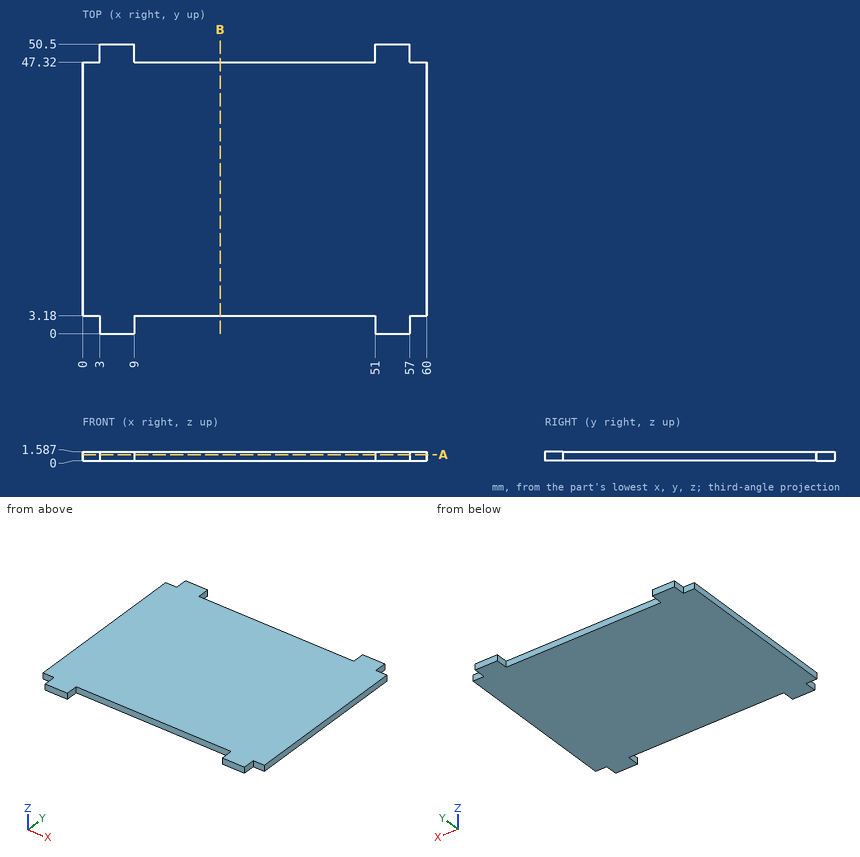
The figure shows three views and two pictorial views of one solid part (mm, origin at its lowest corner). Answer the questions. Give positions to 0.01 mm unless a question says otherwise; leave off trailing zeros. Write each loop counter-clockwise with the first axis right and the second up, starting at its lowest first coordinate (ties: lowest second). Pieces come first, ordered by that corner, then holes. Notation, with made-up numbers: (87.5, 63) - (101.5, 63) arc R25 cw to (101.5, 76) - close; hole circle Ø7 at (89, -33). An arc over 180 degrees is marked (long way). Return JSON: item names as keys, results as strings.
Q1. A cutting plane is placed at B-B, the plane x = 24. Determine the outline of the cut face in (y, z).
Reply:
{"outline": "(3.18, 0) - (47.32, 0) - (47.32, 1.59) - (3.18, 1.59) - close"}
Q2. Given P1, Ø0.5, axis at x = 26.5, z = 0.5, coming from the -Y side; P2, Ø0.5, axis at y = 2.5, z = 1, coming from the -X side; P3, Ø0.5, axis at y = 1.5, z = 1, coming from the +X side, each flat-ended and moving along its own axis, determine where each tip first touches the part or whether it passes through.
Reply:
{"P1": "y = 3.18", "P2": "x = 3", "P3": "x = 57"}
Q3. Consider line 1 along X through (y, z) = (48, 0.45); line 2 along Y through (x, z) = (17.5, 1.05). Determine where each line is inside the solid, lowest interval first. Write a range as [from, to].
Reply:
{"line 1": "[3, 9], [51, 57]", "line 2": "[3.18, 47.32]"}
Q4. A cutting plane is placed at A-A, the plane z = 1.1. Determine the outline of the cut face in (x, y).
Reply:
{"outline": "(0, 3.18) - (3, 3.18) - (3, 0) - (9, 0) - (9, 3.18) - (51, 3.18) - (51, 0) - (57, 0) - (57, 3.18) - (60, 3.18) - (60, 47.32) - (57, 47.32) - (57, 50.5) - (51, 50.5) - (51, 47.32) - (9, 47.32) - (9, 50.5) - (3, 50.5) - (3, 47.32) - (0, 47.32) - close"}
